Read the model definition and answer for the solid it produces. Units are mm, in the model's axes. A direction names the side the tool comes from. Coordinates: 2 decimals unless noted, no trailing zeros. Use CSV: the item, a comma, the result in double quotes.
```python
from build123d import *

# Parameters (mm, degrees)
BOX003_W                  = 500
BOX003_H                  = 500
BOX003_DEPTH              = 500
BOX003_PLACEMENT_ANGLE    = 2
TUBE037_R                 = 85
TUBE037_R_2               = 80
TUBE037_DEPTH             = 19
TUBE036_R                 = 100
TUBE036_R_2               = 80
TUBE036_DEPTH             = 200
PAD034_DEPTH              = 100
PAD035_DEPTH              = 2
COMMON016_PLACEMENT_ANGLE = 38
ARRAY015_COUNT            = 22
ARRAY015_PLACEMENT_ANGLE  = 180
TUBE038_R                 = 34
TUBE038_R_2               = 30
TUBE038_DEPTH             = 19


with BuildPart() as cube003:
    # Box003 → Box003 (new body)
    with BuildSketch(Plane.XY):
        with Locations((250, 250)):
            Rectangle(BOX003_W, BOX003_H)
    extrude(amount=BOX003_DEPTH)


with BuildPart() as cube003_1:
    # Box003 placement: moved
    add(cube003.part.moved(Location((8.73, -250, 0))).rotate(Axis((8.73, -250, 0), (0, 0, 1)), BOX003_PLACEMENT_ANGLE))


with BuildPart() as tube037:
    # Tube037 → Tube037 (new body)
    with BuildSketch(Plane.XY.offset(100.5)):
        Circle(TUBE037_R)
        Circle(TUBE037_R_2, mode=Mode.SUBTRACT)
    extrude(amount=TUBE037_DEPTH)


with BuildPart() as tube036:
    # Tube036 → Tube036 (new body)
    with BuildSketch(Plane.XY):
        Circle(TUBE036_R)
        Circle(TUBE036_R_2, mode=Mode.SUBTRACT)
    extrude(amount=TUBE036_DEPTH)


with BuildPart() as body035:
    # Sketch034 → Pad034 (new body)
    with BuildSketch(Plane.XZ):
        Polygon((0, 0), (0, 2), (26, 0.9), (26, 0), align=None)
    extrude(amount=PAD034_DEPTH)


with BuildPart() as body035_1:
    # Body035 placement: moved
    add(body035.part.moved(Location((-5, 0, 5))))


with BuildPart() as cut010:
    # Sketch035 → Pad035 (new body)
    with BuildSketch(Plane.XY):
        Polygon((0, 0), (0, -52), (25.94305, -47.924315), (8.5, 0), align=None)
    extrude(amount=PAD035_DEPTH)


with BuildPart() as cut010_1:
    # Body036 placement: moved
    add(cut010.part.moved(Location((-5, -33, 5))))

    # Common016: intersect Body035
    add(body035_1.part, mode=Mode.INTERSECT)


with BuildPart() as cut010_2:
    # Common016 placement: moved
    add(cut010_1.part.rotate(Axis((0, 0, 0), (0, 1, 0)), COMMON016_PLACEMENT_ANGLE))

    # Array015: Cut010 ×22 about axis
    array015_axis = Axis((0, 0, 0), (0, 0, 1))


with BuildPart() as cut010_3:
    add(cut010_2.part)
    for i in range(1, ARRAY015_COUNT):
        add(cut010_2.part.rotate(array015_axis, i * 360 / ARRAY015_COUNT))


with BuildPart() as cut010_4:
    # Array015 placement: moved
    add(cut010_3.part.moved(Location((0, 0, 110))).rotate(Axis((0, 0, 110), (0, 1, 0)), ARRAY015_PLACEMENT_ANGLE))

    # Cut010: cut Tube036
    add(tube036.part, mode=Mode.SUBTRACT)


with BuildPart() as stator1h2:
    # Tube038 → Tube038 (new body)
    with BuildSketch(Plane.XY.offset(100.5)):
        Circle(TUBE038_R)
        Circle(TUBE038_R_2, mode=Mode.SUBTRACT)
    extrude(amount=TUBE038_DEPTH)

    # Fusion017: union Tube037, Cut010
    add(tube037.part)
    add(cut010_4.part)

    # Cut011: cut Cube003
    add(cube003_1.part, mode=Mode.SUBTRACT)


solid = stator1h2.part
```
Item 1: Each of these flat-tipped pins is pushed along its axis until it touches: P1, Ø8, axis at x = -66, y = 0, coming from the -Z side; P2, Ø6, axis at x = -41, y = -28, coming from the +Z side; P3, Ø10, axis at x = -16.5, z = 113, coming from the +Y side. Where does it stop, or does it pass through?
Return value:
P1,"stops at z = 105.68"
P2,"stops at z = 110.44"
P3,"stops at y = 84.22"
Item 2: Straight lines are drawn through the part: line 1 along Y through (x, z) = (-73, 109); line 2 along X through (y, z) = (-59, 104.5); line 3 along X through (y, z) = (61.5, 110.5). For each, find the intervals that lie inside material, in ascending order.
Return value:
line 1,"y = -43.54 to -32.73, -25.82 to -23.13, -3.58 to -1.11, 17.41 to 19.88, 32.73 to 43.54"
line 2,"x = -61.19 to -54.03, -42.67 to -39.2, -21.5 to -18.45, -4 to -1.08"
line 3,"x = -58.67 to -51.16, -29.11 to -26.39, -8.93 to -6.54"
Item 3: A tool of negligible diameter and unlimited length cuts with its end or side. For faces 1 (the flat face through (-42.216, 45.316, 108.813)), 2 (the flat face through (-61.96, -1.26, 107.54)), from which of +Z, -Z, +X, -X, +Y, -Y can it reach the whole face along a straight path? Write none if from no direction.
Return value:
face 1,"+Z"
face 2,"-Z"
Item 4: The mould has two halves that part along X. Classify faces 3 (the flat face through (-56.059, -8.317, 102.205)), 4 (the flat face through (-31, 0, 119.5)), 5 (the flat face through (-3.478, 57.186, 112.843)): +X half, -X half, draft (parallel to the pull), parting line (faces both ways), or undercut.
Return value:
face 3,"undercut"
face 4,"draft"
face 5,"+X half"
